from build123d import *

# Parameters (mm, degrees)
SKETCH2_W           = 32
SKETCH2_H           = 34
SKETCH2_R           = 1.6
BOSS_EXTRUDE1_DEPTH = 2
FILLET1_R           = 1


with BuildPart() as part:
    # Sketch2 → Boss-Extrude1 (new body)
    with BuildSketch(Plane(origin=(0, 0, 0), x_dir=(1, 0, 0), z_dir=(0, 1, 0))):
        Rectangle(SKETCH2_W, SKETCH2_H)
        with Locations(Location((-13.5, 0, 0), (0, 0, 270))):
            Circle(SKETCH2_R, mode=Mode.SUBTRACT)
        with Locations(Location((13.5, 0, 0), (0, 0, 90))):
            Circle(SKETCH2_R, mode=Mode.SUBTRACT)
    extrude(amount=BOSS_EXTRUDE1_DEPTH)

    # Fillet1
    # the kernel refuses this fillet: 1 mm, written as the material it takes off along each edge
    with BuildSketch(Plane(origin=(-15, 1, -16), x_dir=(-1, 0, 0), z_dir=(0, 0, -1))) as fillet1_piece_1_section:
        Polygon((0, 0), (FILLET1_R, 0), (FILLET1_R, FILLET1_R), (0, FILLET1_R), align=None)
    fillet1_piece_1 = extrude(amount=FILLET1_R, mode=Mode.PRIVATE)
    fillet1_piece_1 = fillet1_piece_1 - Plane(origin=(-15, 1, -16), x_dir=(0.7071067811865475, -0.7071067811865475, 0), z_dir=(0, 0, -1)) * Sphere(FILLET1_R, mode=Mode.PRIVATE)
    add(fillet1_piece_1, mode=Mode.SUBTRACT)
    with BuildSketch(Plane(origin=(-15, 1, 16), x_dir=(-1, 0, 0), z_dir=(0, 0, 1))) as fillet1_piece_2_section:
        Polygon((0, 0), (FILLET1_R, 0), (FILLET1_R, -FILLET1_R), (0, -FILLET1_R), align=None)
    fillet1_piece_2 = extrude(amount=FILLET1_R, mode=Mode.PRIVATE)
    fillet1_piece_2 = fillet1_piece_2 - Plane(origin=(-15, 1, 16), x_dir=(0.7071067811865475, -0.7071067811865475, 0), z_dir=(0, 0, 1)) * Sphere(FILLET1_R, mode=Mode.PRIVATE)
    add(fillet1_piece_2, mode=Mode.SUBTRACT)
    with BuildSketch(Plane(origin=(15, 1, 16), x_dir=(1, 0, 0), z_dir=(0, 0, 1))) as fillet1_piece_3_section:
        Polygon((0, 0), (FILLET1_R, 0), (FILLET1_R, FILLET1_R), (0, FILLET1_R), align=None)
    fillet1_piece_3 = extrude(amount=FILLET1_R, mode=Mode.PRIVATE)
    fillet1_piece_3 = fillet1_piece_3 - Plane(origin=(15, 1, 16), x_dir=(-0.7071067811865475, -0.7071067811865475, 0), z_dir=(0, 0, 1)) * Sphere(FILLET1_R, mode=Mode.PRIVATE)
    add(fillet1_piece_3, mode=Mode.SUBTRACT)
    with BuildSketch(Plane(origin=(15, 1, -16), x_dir=(0, 0, -1), z_dir=(1, 0, 0))) as fillet1_piece_4_section:
        Polygon((0, 0), (FILLET1_R, 0), (FILLET1_R, FILLET1_R), (0, FILLET1_R), align=None)
    fillet1_piece_4 = extrude(amount=FILLET1_R, mode=Mode.PRIVATE)
    fillet1_piece_4 = fillet1_piece_4 - Plane(origin=(15, 1, -16), x_dir=(0, -0.7071067811865475, 0.7071067811865475), z_dir=(1, 0, 0)) * Sphere(FILLET1_R, mode=Mode.PRIVATE)
    add(fillet1_piece_4, mode=Mode.SUBTRACT)
    with BuildSketch(Plane(origin=(-16, 2, -16), x_dir=(0, -1, 0), z_dir=(0, 0, 1)), Plane(origin=(16, 2, 16), x_dir=(0, -1, 0), z_dir=(0, 0, -1))) as fillet1_piece_5:
        with BuildLine():
            CenterArc((FILLET1_R, FILLET1_R), FILLET1_R, 180, 90)
            Line((0, FILLET1_R), (0, 0))
            Line((0, 0), (FILLET1_R, 0))
        make_face()
    extrude(amount=32, mode=Mode.SUBTRACT)
    with BuildSketch(Plane(origin=(-15, 2, 17), x_dir=(0, -1, 0), z_dir=(1, 0, 0)), Plane(origin=(15, 2, -17), x_dir=(0, -1, 0), z_dir=(-1, 0, 0))) as fillet1_piece_6:
        with BuildLine():
            CenterArc((FILLET1_R, FILLET1_R), FILLET1_R, 180, 90)
            Line((0, FILLET1_R), (0, 0))
            Line((0, 0), (FILLET1_R, 0))
        make_face()
    extrude(amount=30, mode=Mode.SUBTRACT)
    with BuildSketch(Plane(origin=(16, -2.5, 17), x_dir=(-1, 0, 0), z_dir=(0, 1, 0)), Plane(origin=(-16, -2.5, -17), x_dir=(1, 0, 0), z_dir=(0, 1, 0)), Plane(origin=(16, -2.5, -17), x_dir=(0, 0, 1), z_dir=(0, 1, 0))) as fillet1_piece_7:
        with BuildLine():
            CenterArc((FILLET1_R, -FILLET1_R), FILLET1_R, 90, 90)
            Line((0, -FILLET1_R), (0, 0))
            Line((0, 0), (FILLET1_R, 0))
        make_face()
    extrude(amount=3.5, mode=Mode.SUBTRACT)
    with BuildSketch(Plane(origin=(-16, -2.5, 17), x_dir=(1, 0, 0), z_dir=(0, 1, 0))) as fillet1_piece_8:
        with BuildLine():
            CenterArc((FILLET1_R, FILLET1_R), FILLET1_R, 180, 90)
            Line((0, FILLET1_R), (0, 0))
            Line((0, 0), (FILLET1_R, 0))
        make_face()
    extrude(amount=3.5, mode=Mode.SUBTRACT)


solid = part.part
CAD build for the part. Positions are in the model's coordinates, mm. Coordinates: 2 decimals unless noted, no trailing zeros. Write each loop counter-clockwise with the first axis right and the second up, starting at its lowest first coordinate (ties: lowest second). Pieces come first, ordered by that corner, then holes. Notation, with made-up numbers: M 6.5,13 L 14.5,13 A25 cw 14.5,52 Z; hole C -36.5,55.25 d6. An arc over 180 degrees is marked long. Return JSON: item names as keys, results as strings.
Item 1: Drop a flat-ended pin along its axis: pin 1 Ø3.5 at (x, z) = (-13.5, 0) entering from -Y. Give the stop position or say it passes through.
Findings below:
{"pin 1": "stops at y = 0"}
Item 2: Slice it at A-A, the plane x = -13.5. Write the cut outline in (y, z), and give its area (3 significant figures).
Findings below:
{"outline": "M 0,-17 L 1,-17 A1 ccw 2,-16 L 2,-1.6 L 0,-1.6 Z; M 0,1.6 L 2,1.6 L 2,16 A1 ccw 1,17 L 0,17 Z", "area": "61.2 mm2"}
Item 3: Two-plate mould, pull along X, no slides. Class faces 1 (the flat face through (0, 0, 0)), 2 (the cylindrical face through (11.914, 0.986, 0.208)), 3 (the cylindrical face through (15.715, 0.493, -16.699)): +X half, -X half, draft (parallel to the pull), parting line (faces both ways), or undercut.
Findings below:
{"face 1": "draft", "face 2": "undercut", "face 3": "+X half"}
Item 4: Slice it at B-B, the plane y = 0.5. Write the cut outline in (x, z), and give its area (3 significant figures).
Findings below:
{"outline": "M -16,-16 A1 ccw -15,-17 L 15,-17 A1 ccw 16,-16 L 16,16 A1 ccw 15,17 L -15,17 A1 ccw -16,16 Z; hole C -13.5,0 d3.2; hole C 13.5,0 d3.2", "area": "1,070 mm2"}
Item 5: Slice it at C-C, the plane z = 0. Write the cut outline in (x, y), and give its area (3 significant figures).
Findings below:
{"outline": "M -16,0 L -15.1,0 L -15.1,1.99 A1 ccw -16,1 Z; M -11.9,0 L 11.9,0 L 11.9,2 L -11.9,2 Z; M 15.1,0 L 16,0 L 16,1 A1 ccw 15.1,1.99 Z", "area": "50.8 mm2"}
Item 6: Probe line 1 (X direction, y = 0.5, z = 0); line 2 (Z direction, x = 13.5, y = 0.65); line 3 (X direction, y = 1.6, z = 0). List the from-to ranges inside material, lowest first. Write a range as from..to.
Findings below:
{"line 1": "x = -16..-15.1, -11.9..11.9, 15.1..16", "line 2": "z = -17..-1.6, 1.6..17", "line 3": "x = -15.8..-15.1, -11.9..11.9, 15.1..15.8"}
